from build123d import *

# Parameters (mm, degrees)
SKETCH11_R             = 2.1
VSLOT2040_2040_1_DEPTH = 1220


with BuildPart() as part:
    # Sketch11 → Vslot2040 2040(1) (new body)
    with BuildSketch(Plane(origin=(0, 0, 610), x_dir=(-1, 0, 0), z_dir=(0, 0, -1))):
        with BuildLine():
            Line((5.5, -18.2), (3.607842712, -18.2))
            ThreePointArc((3.607842712, -18.2), (3.423066806, -18.323463314), (3.466421356, -18.541421356))
            Line((3.466421356, -18.541421356), (4.925, -20))
            Line((4.925, -20), (9, -20))
            ThreePointArc((9, -20), (9.707106781, -19.707106781), (10, -19))
            Line((10, -19), (10, -14.925))
            Line((10, -14.925), (8.541421356, -13.466421356))
            ThreePointArc((8.541421356, -13.466421356), (8.323463314, -13.423066806), (8.2, -13.607842712))
            Line((8.2, -13.607842712), (8.2, -15.5))
            Line((8.2, -15.5), (6.275, -15.5))
            Line((6.275, -15.5), (3.9, -13.125))
            Line((3.9, -13.125), (3.9, -6.875))
            Line((3.9, -6.875), (6.275, -4.5))
            Line((6.275, -4.5), (8.2, -4.5))
            Line((8.2, -4.5), (8.2, -6.392157288))
            ThreePointArc((8.2, -6.392157288), (8.323463314, -6.576933194), (8.541421356, -6.533578644))
            Line((8.541421356, -6.533578644), (10, -5.075))
            Line((10, -5.075), (10, 5.075))
            Line((10, 5.075), (8.541421356, 6.533578644))
            ThreePointArc((8.541421356, 6.533578644), (8.323463314, 6.576933194), (8.2, 6.392157288))
            Line((8.2, 6.392157288), (8.2, 4.5))
            Line((8.2, 4.5), (6.275, 4.5))
            Line((6.275, 4.5), (3.9, 6.875))
            Line((3.9, 6.875), (3.9, 13.125))
            Line((3.9, 13.125), (6.275, 15.5))
            Line((6.275, 15.5), (8.2, 15.5))
            Line((8.2, 15.5), (8.2, 13.607842712))
            ThreePointArc((8.2, 13.607842712), (8.323463314, 13.423066806), (8.541421356, 13.466421356))
            Line((8.541421356, 13.466421356), (10, 14.925))
            Line((10, 14.925), (10, 19))
            ThreePointArc((10, 19), (9.707106781, 19.707106781), (9, 20))
            Line((9, 20), (4.925, 20))
            Line((4.925, 20), (3.466421356, 18.541421356))
            ThreePointArc((3.466421356, 18.541421356), (3.423066806, 18.323463314), (3.607842712, 18.2))
            Line((3.607842712, 18.2), (5.5, 18.2))
            Line((5.5, 18.2), (5.5, 16.275))
            Line((5.5, 16.275), (3.125, 13.9))
            Line((3.125, 13.9), (-3.125, 13.9))
            Line((-3.125, 13.9), (-5.5, 16.275))
            Line((-5.5, 16.275), (-5.5, 18.2))
            Line((-5.5, 18.2), (-3.607842712, 18.2))
            ThreePointArc((-3.607842712, 18.2), (-3.423066806, 18.323463314), (-3.466421356, 18.541421356))
            Line((-3.466421356, 18.541421356), (-4.925, 20))
            Line((-4.925, 20), (-9, 20))
            ThreePointArc((-9, 20), (-9.707106781, 19.707106781), (-10, 19))
            Line((-10, 19), (-10, 14.925))
            Line((-10, 14.925), (-8.541421356, 13.466421356))
            ThreePointArc((-8.541421356, 13.466421356), (-8.323463314, 13.423066806), (-8.2, 13.607842712))
            Line((-8.2, 13.607842712), (-8.2, 15.5))
            Line((-8.2, 15.5), (-6.275, 15.5))
            Line((-6.275, 15.5), (-3.9, 13.125))
            Line((-3.9, 13.125), (-3.9, 6.875))
            Line((-3.9, 6.875), (-6.275, 4.5))
            Line((-6.275, 4.5), (-8.2, 4.5))
            Line((-8.2, 4.5), (-8.2, 6.392157288))
            ThreePointArc((-8.2, 6.392157288), (-8.323463314, 6.576933194), (-8.541421356, 6.533578644))
            Line((-8.541421356, 6.533578644), (-10, 5.075))
            Line((-10, 5.075), (-10, -5.075))
            Line((-10, -5.075), (-8.541421356, -6.533578644))
            ThreePointArc((-8.541421356, -6.533578644), (-8.323463314, -6.576933194), (-8.2, -6.392157288))
            Line((-8.2, -6.392157288), (-8.2, -4.5))
            Line((-8.2, -4.5), (-6.275, -4.5))
            Line((-6.275, -4.5), (-3.9, -6.875))
            Line((-3.9, -6.875), (-3.9, -13.125))
            Line((-3.9, -13.125), (-6.275, -15.5))
            Line((-6.275, -15.5), (-8.2, -15.5))
            Line((-8.2, -15.5), (-8.2, -13.607842712))
            ThreePointArc((-8.2, -13.607842712), (-8.323463314, -13.423066806), (-8.541421356, -13.466421356))
            Line((-8.541421356, -13.466421356), (-10, -14.925))
            Line((-10, -14.925), (-10, -19))
            ThreePointArc((-10, -19), (-9.707106781, -19.707106781), (-9, -20))
            Line((-9, -20), (-4.925, -20))
            Line((-4.925, -20), (-3.466421356, -18.541421356))
            ThreePointArc((-3.466421356, -18.541421356), (-3.423066806, -18.323463314), (-3.607842712, -18.2))
            Line((-3.607842712, -18.2), (-5.5, -18.2))
            Line((-5.5, -18.2), (-5.5, -16.275))
            Line((-5.5, -16.275), (-3.125, -13.9))
            Line((-3.125, -13.9), (3.125, -13.9))
            Line((3.125, -13.9), (5.5, -16.275))
            Line((5.5, -16.275), (5.5, -18.2))
        make_face()
        with Locations((0, -10)):
            Circle(SKETCH11_R, mode=Mode.SUBTRACT)
        with Locations((0, 10)):
            Circle(SKETCH11_R, mode=Mode.SUBTRACT)
        Polygon((3.125, 6.1), (6.275, 2.95), (8.2, 2.95), (8.2, -2.95), (6.275, -2.95), (3.125, -6.1), (-3.125, -6.1), (-6.275, -2.95), (-8.2, -2.95), (-8.2, 2.95), (-6.275, 2.95), (-3.125, 6.1), align=None, mode=Mode.SUBTRACT)
    extrude(amount=VSLOT2040_2040_1_DEPTH)


solid = part.part
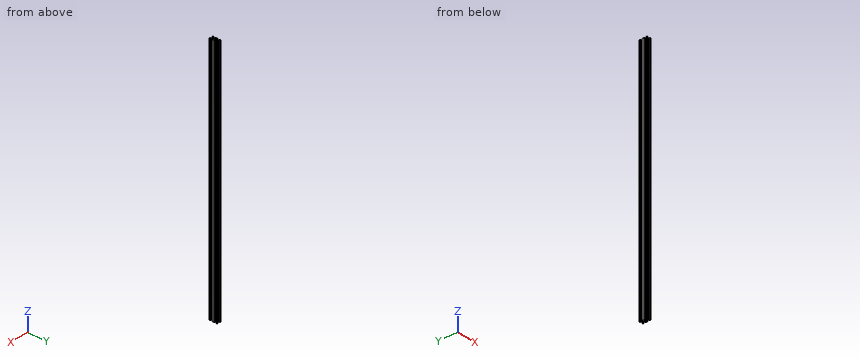
Design review of the part built by this model. Coordinates are the model's own, in mm. Round coordinates to 2 decimals unless told otherwise and drop trailing zeros. One line per question, with ' | ' between items.
1. We need section A-A, the plane z = 249.5. State how many separate pieces and enclosed holes the cut face has, and give its area (3 significant figures).
Results are:
separate pieces: 1 | enclosed holes: 3 | area: 278 mm²
2. For L1, parallel to X at y = -6, z = 364.5 (3 decimals); L2, parallel to Y at x = 0, z = -59.5; L3, parallel to Y at x = 8.75, z = 525 (3 decimals), list the stretches that pass through material, from the lowest coordinate up. Write a range as [from, to].
Results are:
L1: x = [-9.075, -8.2], [-4.775, -3.225], [3.225, 4.775], [8.2, 9.075] | L2: y = [-13.9, -12.1], [-7.9, -6.1], [6.1, 7.9], [12.1, 13.9] | L3: y = [-20, -13.675], [-6.325, 6.325], [13.675, 20]
3. Clearance check with flat-ended pins moving along their axes: P1, Ø7, axis at y = -9, z = -190.5, coming from the +X side (3 decimals); P2, Ø1.9, axis at y = -11, z = 61.5, coming from the -X side; P3, Ø2, axis at x = 0, z = 300, coming from the +Y side. State where each tip first meets the part, or that it passes through.
Results are:
P1: stops at x = 9.575 | P2: stops at x = -3.9 | P3: stops at y = 13.9
